from build123d import *

# Parameters (mm, degrees)
SKETCH1_R           = 2
SKETCH1_R_2         = 1.230505914
SKETCH1_R_3         = 1.065619784
SKETCH1_R_4         = 2.013222478
SKETCH1_R_5         = 0.813520941
BOSS_EXTRUDE1_DEPTH = 1.6


with BuildPart() as part:
    # Sketch1 → Boss-Extrude1 (new body)
    with BuildSketch(Plane.XY):
        with BuildLine():
            Line((-43.390980767, 89.104719312), (-43.390980767, 0.289327535))
            Line((-43.390980767, 0.289327535), (-16.705853066, 0.289327535))
            Line((-16.705853066, 0.289327535), (-16.705853066, 55.060343389))
            ThreePointArc((-16.705853066, 55.060343389), (-12.260853066, 57.261941316), (-7.815853066, 55.060343389))
            Line((-7.815853066, 55.060343389), (-7.815853066, 47.714452921))
            Line((-7.815853066, 47.714452921), (66.454194778, 47.714452921))
            Line((66.454194778, 47.714452921), (66.454194778, 48.476452921))
            Line((66.454194778, 48.476452921), (66.454194778, 89.104719312))
            Line((66.454194778, 89.104719312), (43.055141469, 89.104719312))
            Line((43.055141469, 89.104719312), (43.055141469, 77.440236178))
            Line((43.055141469, 77.440236178), (22.130034422, 77.440236178))
            Line((22.130034422, 77.440236178), (22.130034422, 89.104719312))
            Line((22.130034422, 89.104719312), (-43.390980767, 89.104719312))
        make_face()
        with Locations((-30.204884299, 3.786024021)):
            Circle(SKETCH1_R, mode=Mode.SUBTRACT)
        with Locations((-35.12092244, 16.959583239)):
            Circle(SKETCH1_R_2, mode=Mode.SUBTRACT)
        with Locations((-33.844684508, 19.525695646)):
            Circle(SKETCH1_R_3, mode=Mode.SUBTRACT)
        with Locations((-30.03593296, 16.959583239)):
            Circle(SKETCH1_R_4, mode=Mode.SUBTRACT)
        with Locations((-25.002523415, 16.959583239)):
            Circle(SKETCH1_R_2, mode=Mode.SUBTRACT)
        with Locations((-27.486377969, 22.058201664)):
            Circle(SKETCH1_R_3, mode=Mode.SUBTRACT)
        with Locations((-35.12092244, 38.997647894)):
            Circle(SKETCH1_R_2, mode=Mode.SUBTRACT)
        with Locations((-30.03593296, 38.997647894)):
            Circle(SKETCH1_R_4, mode=Mode.SUBTRACT)
        with Locations((-33.844684508, 41.478225078)):
            Circle(SKETCH1_R_3, mode=Mode.SUBTRACT)
        with Locations((-25.002523415, 38.997647894)):
            Circle(SKETCH1_R_2, mode=Mode.SUBTRACT)
        with Locations((-27.486377969, 44.045488268)):
            Circle(SKETCH1_R_3, mode=Mode.SUBTRACT)
        with Locations((3.702023102, 52.815358714)):
            Circle(SKETCH1_R_5, mode=Mode.SUBTRACT)
        with Locations((6.270118325, 52.815358714)):
            Circle(SKETCH1_R_5, mode=Mode.SUBTRACT)
        with Locations((-39.919519396, 85.68551268)):
            Circle(SKETCH1_R, mode=Mode.SUBTRACT)
        with Locations((11.611877913, 52.793786064)):
            Circle(SKETCH1_R_5, mode=Mode.SUBTRACT)
        with Locations((14.144190439, 52.793786064)):
            Circle(SKETCH1_R_5, mode=Mode.SUBTRACT)
        with Locations((19.502215653, 52.793786064)):
            Circle(SKETCH1_R_5, mode=Mode.SUBTRACT)
        with Locations((22.036775121, 52.793786064)):
            Circle(SKETCH1_R_5, mode=Mode.SUBTRACT)
        with Locations((27.392356576, 52.793786064)):
            Circle(SKETCH1_R_5, mode=Mode.SUBTRACT)
        with Locations((29.931743714, 52.793786064)):
            Circle(SKETCH1_R_5, mode=Mode.SUBTRACT)
        with Locations((35.282808648, 52.828198648)):
            Circle(SKETCH1_R_5, mode=Mode.SUBTRACT)
        with Locations((37.828059634, 52.828198648)):
            Circle(SKETCH1_R_5, mode=Mode.SUBTRACT)
        with Locations((22.130034422, 60.797517772)):
            Circle(SKETCH1_R, mode=Mode.SUBTRACT)
        with Locations((43.190352962, 52.793786064)):
            Circle(SKETCH1_R_5, mode=Mode.SUBTRACT)
        with Locations((45.720365379, 52.828198648)):
            Circle(SKETCH1_R_5, mode=Mode.SUBTRACT)
        with Locations((51.055737978, 52.793786064)):
            Circle(SKETCH1_R_5, mode=Mode.SUBTRACT)
        with Locations((53.630473203, 52.793786064)):
            Circle(SKETCH1_R_5, mode=Mode.SUBTRACT)
        with Locations((58.949894198, 52.793786064)):
            Circle(SKETCH1_R_5, mode=Mode.SUBTRACT)
        with Locations((61.501156091, 52.793786064)):
            Circle(SKETCH1_R_5, mode=Mode.SUBTRACT)
        with Locations((43.125719502, 60.797517772)):
            Circle(SKETCH1_R, mode=Mode.SUBTRACT)
        with Locations((22.130034422, 73.370517772)):
            Circle(SKETCH1_R, mode=Mode.SUBTRACT)
        with Locations((18.59384388, 85.577256227)):
            Circle(SKETCH1_R, mode=Mode.SUBTRACT)
        with Locations((43.125719502, 73.370517772)):
            Circle(SKETCH1_R, mode=Mode.SUBTRACT)
        with Locations((62.904421424, 85.577256227)):
            Circle(SKETCH1_R, mode=Mode.SUBTRACT)
    extrude(amount=BOSS_EXTRUDE1_DEPTH)


solid = part.part
Check sheet for the modelled part. Datum: model origin and axes. Units: mm. Round coordinates to 2 decimals unless told otherwise and drop trailing zeros. Order: outer loops, then holes, each group sorted by start corner. A loop starts at its lowest first (then second) coordinate and runs counter-clockwise, first axis right, second up.
(1) Go/stop test with a flat-tipped pin: P1, Ø2.5, axis at x = 43.19, y = 52.79, coming from the -Z side. Record where the tip stops, or that it passes through.
(2) Cross-section at C-C, the plane z = 0.35. State how many separate pieces and enclosed holes the cut face has, and give its area (3 significant figures).
(3) Cross-section at B-B, the plane y = 30. Enter the section's corners in (x, z).
(4) Cross-section at A-A, the plane x = -25. Enter the section's corners in (y, z).
(5) Draft check along X on faces 1 (the cylindrical face through (42.87, 62.78, 0.79)), 2 (the flat face through (-1, 55, 0)). Enter one of: pulls with the +X half, pulls with the -X half, needs draft (parallel to the pull), parting line crosses it, or undercut.
(6) Scan lines: probe 1 along X at (y, z) = (17, 1.45); probe 2 along X at (y, z) = (78, 1.25); probe 3 along Y at (x, z) = (27.5, 0.3). Record each from-to range of solid material in increasing order.
Check sheet entries:
1. P1: stops at z = 0
2. separate pieces: 1
2. enclosed holes: 34
2. area: 5,300 mm2
3. outline: (-43.39, 0) - (-16.71, 0) - (-16.71, 1.6) - (-43.39, 1.6) - close
4. outline: (0.29, 0) - (15.73, 0) - (15.73, 1.6) - (0.29, 1.6) - close; (18.19, 0) - (37.77, 0) - (37.77, 1.6) - (18.19, 1.6) - close; (40.23, 0) - (89.1, 0) - (89.1, 1.6) - (40.23, 1.6) - close
5. face 1: undercut
5. face 2: needs draft
6. probe 1: x = -43.39 to -36.35, -33.89 to -32.05, -28.02 to -26.23, -23.77 to -16.71
6. probe 2: x = -43.39 to 22.13, 43.06 to 66.45
6. probe 3: y = 47.71 to 51.99, 53.6 to 77.44
